Geometry check sheet. Reference: the model listing, model coordinates, mm. A direction names the side the tool comes from. Round coordinates to 2 decimals unless told otherwise and drop trailing zeros. Order: outer loops, then holes, each group sorted by start corner. A loop starts at its lowest first (then second) coordinate and runs counter-clockwise, first axis right, second up. Notation, with made-up numbers: (53, -35.5) -> (108, -35.5) arc R13 cw to (108, -12.5) -> close; hole circle Ø5 at (55, -6). An arc over 180 degrees is marked (long way). Use a Markdown table: item, result. Add a question column.
Item 1: Sectioned sample at B-B, the plane x = 2. Record the cut outline in (y, z).
Item 2: Sectioned sample at C-C, the plane z = 10. Record the cut outline in (x, y), and give its area (3 significant figures).
Item 3: Mould release check, pull along X, two halves, no side actions. Record for faces 4 (the cylindrical face through (11.5, 1.5, 10.1)), 5 (the flat face through (-38.4, 8, -30.6)), 6 (the cylindrical face through (33.5, 1.5, 24.9)): pulls with the +X half, pulls with the -X half, needs draft (parallel to the pull), parting line crosses it, or undercut.
Item 4: Gauge pin test, flat ends, axial feed: pin 1 Ø5 at (x, z) = (-12.5, -25.5) entering from +Y; pin 2 Ø2.5 at (x, z) = (-37.5, 31.5) entering from -Y. Record the tip position at first contact, or that the pin passes through.
Item 5: Set-up check for faces 1 (the cylindrical face through (-34.5, 1.5, -21.4)), 2 (the cylindrical face through (-35.726, 5.535, 30.577)), 3 (the flat face through (18, 8, 27)): record each of +Z, -Z, +X, -X, +Y, -Y from which the full face is reachable in a straight line by a thin tool's end or side.
Item 6: Material ranges on probe 1 along Z at (x, y) = (-9, 2.75); probe 2 along Z at (x, y) = (-37, 5.75); probe 3 along Y at (x, z) = (-2, -26), recorded low to high. Write a range as [from, to].
Item 7: Sectioned sample at D-D, the plane z = -27.5. Record the cut outline in (x, y), and give its area (3 significant figures).
Item 8: Sectioned sample at A-A, the plane y = 4.75. Record the cut outline in (x, z), and give its area (3 significant figures).
from build123d import *

# Parameters (mm, degrees)
ESBO_O1_W                = 95
ESBO_O1_H                = 69
RESSALTO_EXTRUS_O1_DEPTH = 3
ESBO_O2_R                = 13.9
CORTE_EXTRUS_O1_DEPTH    = 59.783501087
ESBO_O4_R                = 1
CORTE_EXTRUS_O2_DEPTH    = 59.783501087
RESSALTO_EXTRUS_O2_START = 5
ESBO_O5_R                = 2
ESBO_O5_R_2              = 1
RESSALTO_EXTRUS_O2_DEPTH = 5
FILETE1_R                = 40
FILETE2_R                = 10
CORTE_EXTRUS_O3_DEPTH    = 59.919436521


with BuildPart() as part:
    # Esboço1 → Ressalto-extrusão1 (new body)
    with BuildSketch(Plane(origin=(0, 0, 0), x_dir=(1, 0, 0), z_dir=(0, 1, 0))):
        Rectangle(ESBO_O1_W, ESBO_O1_H)
    extrude(amount=RESSALTO_EXTRUS_O1_DEPTH)

    # Esboço2 → Corte-extrusão1 (cut, through all)
    with BuildSketch(Plane(origin=(0, 3, 0), x_dir=(1, 0, 0), z_dir=(0, 1, 0))):
        with Locations(Location((30.6, 0, 0), (0, 0, 270))):
            Circle(ESBO_O2_R)
    extrude(amount=-CORTE_EXTRUS_O1_DEPTH, mode=Mode.SUBTRACT)

    # Esboço4 → Corte-extrusão2 (cut, through all)
    with BuildSketch(Plane(origin=(0, 3, 0), x_dir=(1, 0, 0), z_dir=(0, 1, 0))):
        with Locations(Location((16.7, 27.5, 0), (0, 0, 270))):
            Circle(ESBO_O4_R)
        with Locations(Location((16.7, -27.5, 0), (0, 0, 90))):
            Circle(ESBO_O4_R)
        with Locations(Location((-37.5, 31.5, 0), (0, 0, 270))):
            Circle(ESBO_O4_R)
        with Locations(Location((-37.5, -31.5, 0), (0, 0, 90))):
            Circle(ESBO_O4_R)
    extrude(amount=-CORTE_EXTRUS_O2_DEPTH, mode=Mode.SUBTRACT)

    # Esboço5 → Ressalto-extrusão2 (add)
    # profile 1 of 4: a face of its own
    with BuildSketch(Plane(origin=(0, 3, 0), x_dir=(1, 0, 0), z_dir=(0, 1, 0)).offset(RESSALTO_EXTRUS_O2_START)):
        with Locations(Location((-37.5, 31.5, 0), (0, 0, 270))):
            Circle(ESBO_O5_R)
        with Locations(Location((-37.5, 31.5, 0), (0, 0, 270))):
            Circle(ESBO_O5_R_2, mode=Mode.SUBTRACT)
    # profile 2 of 4: a face of its own
    with BuildSketch(Plane(origin=(0, 3, 0), x_dir=(1, 0, 0), z_dir=(0, 1, 0)).offset(RESSALTO_EXTRUS_O2_START)):
        with Locations(Location((16.7, 27.5, 0), (0, 0, 270))):
            Circle(ESBO_O5_R)
        with Locations(Location((16.7, 27.5, 0), (0, 0, 270))):
            Circle(ESBO_O5_R_2, mode=Mode.SUBTRACT)
    # profile 3 of 4: a face of its own
    with BuildSketch(Plane(origin=(0, 3, 0), x_dir=(1, 0, 0), z_dir=(0, 1, 0)).offset(RESSALTO_EXTRUS_O2_START)):
        with Locations(Location((16.7, -27.5, 0), (0, 0, 90))):
            Circle(ESBO_O5_R)
        with Locations(Location((16.7, -27.5, 0), (0, 0, 90))):
            Circle(ESBO_O5_R_2, mode=Mode.SUBTRACT)
    # profile 4 of 4: a face of its own
    with BuildSketch(Plane(origin=(0, 3, 0), x_dir=(1, 0, 0), z_dir=(0, 1, 0)).offset(RESSALTO_EXTRUS_O2_START)):
        with Locations(Location((-37.5, -31.5, 0), (0, 0, 90))):
            Circle(ESBO_O5_R)
        with Locations(Location((-37.5, -31.5, 0), (0, 0, 90))):
            Circle(ESBO_O5_R_2, mode=Mode.SUBTRACT)
    extrude(amount=-RESSALTO_EXTRUS_O2_DEPTH)

    # Filete1
    # the kernel refuses this fillet: 40 mm, written as the material it takes off along each edge
    with BuildSketch(Plane(origin=(47.5, -100, -34.5), x_dir=(-1, 0, 0), z_dir=(0, 1, 0))) as filete1_piece_1:
        with BuildLine():
            CenterArc((FILETE1_R, FILETE1_R), FILETE1_R, 180, 90)
            Line((0, FILETE1_R), (0, 0))
            Line((0, 0), (FILETE1_R, 0))
        make_face()
    extrude(amount=203, mode=Mode.SUBTRACT)
    with BuildSketch(Plane(origin=(47.5, -100, 34.5), x_dir=(-1, 0, 0), z_dir=(0, 1, 0))) as filete1_piece_2:
        with BuildLine():
            CenterArc((FILETE1_R, -FILETE1_R), FILETE1_R, 90, 90)
            Line((0, -FILETE1_R), (0, 0))
            Line((0, 0), (FILETE1_R, 0))
        make_face()
    extrude(amount=203, mode=Mode.SUBTRACT)

    # Filete2
    filete2_edges = [part.edges().sort_by_distance(p)[0] for p in [
        (-47.5, 1.5, 34.5),
        (-47.5, 1.5, -34.5),
    ]]
    fillet(filete2_edges, radius=FILETE2_R)

    # Esboço7 → Corte-extrusão3 (cut, through all)
    with BuildSketch(Plane(origin=(0, 3, 0), x_dir=(1, 0, 0), z_dir=(0, 1, 0))):
        with BuildLine():
            Line((-31.5, 13), (8.5, 13))
            ThreePointArc((8.5, 13), (11.5, 10), (8.5, 7))
            Line((8.5, 7), (-31.5, 7))
            ThreePointArc((-31.5, 7), (-34.5, 10), (-31.5, 13))
        make_face()
        with BuildLine():
            Line((-31.5, 24.5), (8.5, 24.5))
            ThreePointArc((8.5, 24.5), (11.5, 21.5), (8.5, 18.5))
            Line((8.5, 18.5), (-31.5, 18.5))
            ThreePointArc((-31.5, 18.5), (-34.5, 21.5), (-31.5, 24.5))
        make_face()
        with BuildLine():
            Line((-31.5, -24.5), (8.5, -24.5))
            ThreePointArc((8.5, -24.5), (11.5, -21.5), (8.5, -18.5))
            Line((8.5, -18.5), (-31.5, -18.5))
            ThreePointArc((-31.5, -18.5), (-34.5, -21.5), (-31.5, -24.5))
        make_face()
        with BuildLine():
            Line((-31.5, -13), (8.5, -13))
            ThreePointArc((8.5, -13), (11.5, -10), (8.5, -7))
            Line((8.5, -7), (-31.5, -7))
            ThreePointArc((-31.5, -7), (-34.5, -10), (-31.5, -13))
        make_face()
    extrude(amount=-CORTE_EXTRUS_O3_DEPTH, mode=Mode.SUBTRACT)


solid = part.part
Found:
| question | item | result |
|---|---|---|
| 1 | outline | (0, -34.5) -> (3, -34.5) -> (3, -24.5) -> (0, -24.5) -> close; (0, -18.5) -> (3, -18.5) -> (3, -13) -> (0, -13) -> close; (0, -7) -> (3, -7) -> (3, 7) -> (0, 7) -> close; (0, 13) -> (3, 13) -> (3, 18.5) -> (0, 18.5) -> close; (0, 24.5) -> (3, 24.5) -> (3, 34.5) -> (0, 34.5) -> close |
| 2 | outline | (-47.5, 0) -> (-34.5, 0) -> (-34.5, 3) -> (-47.5, 3) -> close; (11.5, 0) -> (20.95, 0) -> (20.95, 3) -> (11.5, 3) -> close; (40.25, 0) -> (44.37, 0) -> (44.37, 3) -> (40.25, 3) -> close |
| 2 | area | 79.7 mm2 |
| 3 | face 4 | undercut |
| 3 | face 5 | needs draft |
| 3 | face 6 | pulls with the +X half |
| 4 | pin 1 | stops at y = 3 |
| 4 | pin 2 | stops at y = 0 |
| 5 | face 1 | +Y, -Y |
| 5 | face 2 | +Y |
| 5 | face 3 | +Z, -Z, +X, -X, +Y |
| 6 | probe 1 | z = [-34.5, -24.5], [-18.5, -13], [-7, 7], [13, 18.5], [24.5, 34.5] |
| 6 | probe 2 | z = [-33.44, -32.37], [-30.63, -29.56], [29.56, 30.63], [32.37, 33.44] |
| 6 | probe 3 | y = [0, 3] |
| 7 | outline | (-47.04, 0) -> (15.7, 0) -> (15.7, 8) -> (14.7, 8) -> (14.7, 3) -> (-47.04, 3) -> close; (17.7, 0) -> (30.11, 0) -> (30.11, 3) -> (18.7, 3) -> (18.7, 8) -> (17.7, 8) -> close |
| 7 | area | 235 mm2 |
| 8 | outline | circle Ø4 at (-37.5, -31.5); circle Ø4 at (-37.5, 31.5); circle Ø4 at (16.7, -27.5); circle Ø4 at (16.7, 27.5); hole circle Ø2 at (-37.5, -31.5); hole circle Ø2 at (-37.5, 31.5); hole circle Ø2 at (16.7, -27.5); hole circle Ø2 at (16.7, 27.5) |
| 8 | area | 37.7 mm2 |
